from build123d import *

# Parameters (mm, degrees)
SKETCH1_W                      = 163
SKETCH1_H                      = 119.634
BOSS_EXTRUDE1_DEPTH            = 3.175
SKETCH2_R                      = 2.286
CUT_EXTRUDE1_DEPTH             = 102.145460175
MIRROR2_COPY_1_SKETCH_R        = 2.286
MIRROR2_COPY_1_DEPTH           = 102.145460175
SKETCH3_R                      = 10
CUT_EXTRUDE2_DEPTH             = 102.145460175
F_1_16_0_0625_DIAMETER_HOLE1_D = 6.35


with BuildPart() as part:
    # Sketch1 → Boss-Extrude1 (new body)
    with BuildSketch(Plane(origin=(0, 0, 0), x_dir=(1, 0, 0), z_dir=(0, 1, 0))):
        Rectangle(SKETCH1_W, SKETCH1_H)
    extrude(amount=BOSS_EXTRUDE1_DEPTH)

    # Sketch2 → Cut-Extrude1 (cut, through all)
    with BuildSketch(Plane(origin=(0, 3.175, 0), x_dir=(1, 0, 0), z_dir=(0, 1, 0))):
        with Locations(Location((72.61, -51.7398, 0), (0, 0, 270))):
            Circle(SKETCH2_R)
        with Locations(Location((48.61, -51.7398, 0), (0, 0, 270))):
            Circle(SKETCH2_R)
        with Locations(Location((48.61, -30.3398, 0), (0, 0, 270))):
            Circle(SKETCH2_R)
        with Locations(Location((72.61, -30.3398, 0), (0, 0, 270))):
            Circle(SKETCH2_R)
    cut_extrude1 = extrude(amount=-CUT_EXTRUDE1_DEPTH, mode=Mode.SUBTRACT)

    # Mirror1: Cut-Extrude1 across plane
    add(cut_extrude1.mirror(Plane.XY), mode=Mode.SUBTRACT)

    # Mirror2: Cut-Extrude1 across plane
    add(cut_extrude1.mirror(Plane(origin=(0, 0, 0), x_dir=(0, 0, 1), z_dir=(1, 0, 0))), mode=Mode.SUBTRACT)

    # Mirror2 copy 1 sketch → Mirror2 copy 1 (cut, through all)
    with BuildSketch(Plane(origin=(0, 3.175, 0), x_dir=(-1, 0, 0), z_dir=(0, 1, 0))):
        with Locations(Location((72.61, -51.7398, 0), (0, 0, 270))):
            Circle(MIRROR2_COPY_1_SKETCH_R)
        with Locations(Location((48.61, -51.7398, 0), (0, 0, 270))):
            Circle(MIRROR2_COPY_1_SKETCH_R)
        with Locations(Location((48.61, -30.3398, 0), (0, 0, 270))):
            Circle(MIRROR2_COPY_1_SKETCH_R)
        with Locations(Location((72.61, -30.3398, 0), (0, 0, 270))):
            Circle(MIRROR2_COPY_1_SKETCH_R)
    extrude(amount=-MIRROR2_COPY_1_DEPTH, mode=Mode.SUBTRACT)

    # Sketch3 → Cut-Extrude2 (cut, through all)
    with BuildSketch(Plane(origin=(0, 3.175, 0), x_dir=(1, 0, 0), z_dir=(0, 1, 0))):
        with Locations(Location((0, 0, 0), (0, 0, 270))):
            Circle(SKETCH3_R)
    extrude(amount=-CUT_EXTRUDE2_DEPTH, mode=Mode.SUBTRACT)

    # 1/16 (0.0625) Diameter Hole1 (through all)
    with Locations(Plane(origin=(0, 3.175, 0), x_dir=(1, 0, 0), z_dir=(0, 1, 0))):
        with Locations((-10, -50), (10, -50)):
            Hole(F_1_16_0_0625_DIAMETER_HOLE1_D / 2)


solid = part.part
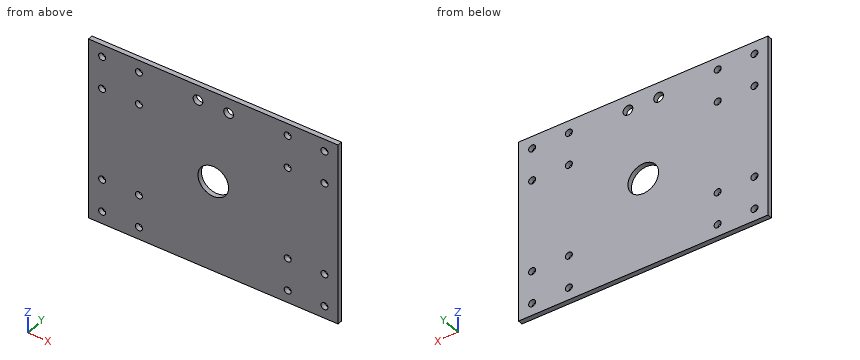
Work out the finished part from the listing and answer in its coordinate system (mm). Round coordinates to 2 decimals unless told otherwise and drop trailing zeros. Write each loop counter-clockwise with the first axis right and the second up, starting at its lowest first coordinate (ties: lowest second). Pieces come first, ordered by that corner, then holes.
1) A cutting plane is placed at C-C (x = -48.61). Give the vertices of the cut face in (y, z) (3 decimals).
2) Straight lines are drawn through the part: line 1 (Z direction, x = -48.61, y = 2); line 2 (X direction, y = 0.2, z = 48); line 3 (X direction, y = 2, z = 5.5). For each, find the intervals that lie inside material, in ascending order.
3) A cutting plane is placed at B-B (x = 0). Give the vertices of the cut face in (y, z) (3 decimals).
4) A cutting plane is placed at A-A (z = 0). Give the vertices of the cut face in (x, y) (3 decimals), plus the area to 3 significant figures.
5) A cutting plane is placed at D-D (y = 0.55). Give the number of separate pieces and of enclosed holes in the cut face, plus the area to 3 significant figures.
Completed:
1. outline: (0, -59.817) - (3.175, -59.817) - (3.175, -54.026) - (0, -54.026) - close; (0, -49.454) - (3.175, -49.454) - (3.175, -32.626) - (0, -32.626) - close; (0, -28.054) - (3.175, -28.054) - (3.175, 28.054) - (0, 28.054) - close; (0, 32.626) - (3.175, 32.626) - (3.175, 49.454) - (0, 49.454) - close; (0, 54.026) - (3.175, 54.026) - (3.175, 59.817) - (0, 59.817) - close
2. line 1: z = -59.82 to -54.03, -49.45 to -32.63, -28.05 to 28.05, 32.63 to 49.45, 54.03 to 59.82
2. line 2: x = -81.5 to -12.47, -7.53 to 7.53, 12.47 to 81.5
2. line 3: x = -81.5 to -8.35, 8.35 to 81.5
3. outline: (0, -59.817) - (3.175, -59.817) - (3.175, -10) - (0, -10) - close; (0, 10) - (3.175, 10) - (3.175, 59.817) - (0, 59.817) - close
4. outline: (-81.5, 0) - (-10, 0) - (-10, 3.175) - (-81.5, 3.175) - close; (10, 0) - (81.5, 0) - (81.5, 3.175) - (10, 3.175) - close
4. area: 454 mm2
5. separate pieces: 1
5. enclosed holes: 19
5. area: 18,900 mm2
